```python
from build123d import *

# Parameters (mm, degrees)
F1_DEPTH     = 50
F3_DEPTH     = 45
F4_W         = 15
F4_H         = 40
F5_DEPTH     = 20
F6_T1_DEPTH  = 133.8850999909
F6_T3_DEPTH  = 133.8850999909
F6_T5_DEPTH  = 133.8850999909
F6_T10_DEPTH = 133.8850999909
F6_T15_DEPTH = 133.8850999909
F6_T20_DEPTH = 133.8850999909
F6_T25_DEPTH = 133.8850999909
F6_T30_DEPTH = 133.8850999909


# Not quite as in the source:
# - a fillet or chamfer that OpenCascade refuses, or shapes differently, is made with other operations: its cross-section is extruded or revolved along the edge and cut away or added


with BuildPart() as f1:
    # F0 (on Top) → F1 (new body)
    with BuildSketch(Plane.XY):
        Polygon((29.9990277389, 0.2415258118), (14.7903463808, 26.1006830166), (-15.2086813581, 25.8591572049), (-29.9990277389, -0.2415258118), (-14.7903463808, -26.1006830166), (15.2086813581, -25.8591572049), align=None)
    extrude(amount=F1_DEPTH)

    # F2 (on face) → F3 (cut)
    with BuildSketch(Plane.XY.offset(50)):
        Polygon((24.9981357174, 0.3053041981), (12.2346666673, 21.8016726776), (-12.7634690502, 21.4963684795), (-24.9981357174, -0.3053041981), (-12.2346666673, -21.8016726776), (12.7634690502, -21.4963684795), align=None)
    extrude(amount=-F3_DEPTH, mode=Mode.SUBTRACT)

    # F4 (on face) → F5 (join)
    with BuildSketch(Plane(origin=(0.2091674886, -25.9799201108, 0), x_dir=(0.9999675913, 0.0080508604, 0), z_dir=(0.0080508604, -0.9999675913, 0))):
        with Locations((0, 25)):
            Rectangle(F4_W, F4_H)
    extrude(amount=F5_DEPTH)

    # F6: chamfer of 20 x 5 on 6 edges, made by hand

    # F6_s2 → F6_t1 (cut)
    with BuildSketch(Plane(origin=(33.0034500683, 58.2415425919, 0), x_dir=(0, 0, 1), z_dir=(-0.493011546, -0.8700227672, 0))):
        Polygon((50, 20.9807621135), (30, 25.9807621135), (50, 25.9807621135), align=None)
    extrude(amount=F6_T1_DEPTH, mode=Mode.SUBTRACT)

    # F6_s4 → F6_t3 (cut)
    with BuildSketch(Plane(origin=(66.9403804743, 0.5389451243, 0), x_dir=(0, 0, 1), z_dir=(-0.9999675913, -0.0080508604, 0))):
        Polygon((50, 20.9807621135), (30, 25.9807621135), (50, 25.9807621135), align=None)
    extrude(amount=F6_T3_DEPTH, mode=Mode.SUBTRACT)

    # F6_s6 → F6_t5 (cut)
    with BuildSketch(Plane(origin=(33.936930406, -57.7025974676, 0), x_dir=(0, 0, 1), z_dir=(-0.5069560453, 0.8619719068, 0))):
        Polygon((30, 25.9807621135), (50, 20.9807621135), (50, 25.9807621135), align=None)
    extrude(amount=F6_T5_DEPTH, mode=Mode.SUBTRACT)


with BuildPart() as f6_tool8:
    # F6_s9 → F6_t10 (new body)
    with BuildSketch(Plane(origin=(-33.0034500683, -58.2415425919, 0), x_dir=(0, 0, 1), z_dir=(0.493011546, 0.8700227672, 0))):
        Polygon((30, 25.9807621135), (50, 20.9807621135), (50, 25.9807621135), align=None)
    extrude(amount=F6_T10_DEPTH)

    split(bisect_by=Plane(origin=(7.4997569347, 0.0603814529, 0), x_dir=(0, 0, 1), z_dir=(0.9999675913, 0.0080508604, 0)), keep=Keep.TOP)


with BuildPart() as f1_1:
    add(f1.part)

    # F6_t7: cut F6_tool8
    add(f6_tool8.part, mode=Mode.SUBTRACT)


with BuildPart() as f6_tool13:
    # F6_s14 → F6_t15 (new body)
    with BuildSketch(Plane(origin=(-66.9403804743, -0.5389451243, 0), x_dir=(0, 0, 1), z_dir=(0.9999675913, 0.0080508604, 0))):
        Polygon((30, 25.9807621135), (50, 20.9807621135), (50, 25.9807621135), align=None)
    extrude(amount=F6_T15_DEPTH)

    split(bisect_by=Plane(origin=(-7.4997569347, -0.0603814529, 0), x_dir=(0, 0, 1), z_dir=(-0.9999675913, -0.0080508604, 0)), keep=Keep.TOP)


with BuildPart() as f1_2:
    add(f1_1.part)

    # F6_t12: cut F6_tool13
    add(f6_tool13.part, mode=Mode.SUBTRACT)


with BuildPart() as f6_tool18:
    # F6_s19 → F6_t20 (new body)
    with BuildSketch(Plane(origin=(-66.9403804743, -0.5389451243, 0), x_dir=(0, 0, 1), z_dir=(0.9999675913, 0.0080508604, 0))):
        Polygon((30, 25.9807621135), (50, 20.9807621135), (50, 25.9807621135), align=None)
    extrude(amount=F6_T20_DEPTH)

    split(bisect_by=Plane.XY.offset(45), keep=Keep.TOP)


with BuildPart() as f1_3:
    add(f1_2.part)

    # F6_t17: cut F6_tool18
    add(f6_tool18.part, mode=Mode.SUBTRACT)


with BuildPart() as f6_tool23:
    # F6_s24 → F6_t25 (new body)
    with BuildSketch(Plane(origin=(-66.9403804743, -0.5389451243, 0), x_dir=(0, 0, 1), z_dir=(0.9999675913, 0.0080508604, 0))):
        Polygon((30, 25.9807621135), (50, 20.9807621135), (50, 25.9807621135), align=None)
    extrude(amount=F6_T25_DEPTH)

    split(bisect_by=Plane(origin=(7.4997569347, 0.0603814529, 0), x_dir=(0, 0, 1), z_dir=(0.9999675913, 0.0080508604, 0)), keep=Keep.TOP)


with BuildPart() as f1_4:
    add(f1_3.part)

    # F6_t22: cut F6_tool23
    add(f6_tool23.part, mode=Mode.SUBTRACT)


with BuildPart() as f6_tool28:
    # F6_s29 → F6_t30 (new body)
    with BuildSketch(Plane(origin=(-33.936930406, 57.7025974676, 0), x_dir=(0, 0, 1), z_dir=(0.5069560453, -0.8619719068, 0))):
        Polygon((50, 20.9807621135), (30, 25.9807621135), (50, 25.9807621135), align=None)
    extrude(amount=F6_T30_DEPTH)

    split(bisect_by=Plane(origin=(-7.4997569347, -0.0603814529, 0), x_dir=(0, 0, 1), z_dir=(-0.9999675913, -0.0080508604, 0)), keep=Keep.TOP)


with BuildPart() as f1_5:
    add(f1_4.part)

    # F6_t27: cut F6_tool28
    add(f6_tool28.part, mode=Mode.SUBTRACT)


solid = f1_5.part
```
The listing builds one solid part. Answer for the finished solid, in the listing's coordinates (mm). A direction names the side the tool comes from. Give positions to 0.01 mm unless a question says otherwise; leave off trailing zeros. Order: outer loops, then holes, each group sorted by start corner. A loop starts at its lowest first (then second) coordinate and runs counter-clockwise, first axis right, second up. Notation, with made-up numbers: (15, 65.5) - (59, 65.5) arc R10 ccw to (59, 76.5) - close; hole circle Ø8 at (-27.75, 32.5). An arc over 180 degrees is marked (long way). Answer in a Markdown table with one row per item. Add a question column.
Q1. Which of the six approach directions +Z, -Z, +X, -X, +Y, -Y give full straight-line access (tool end or side, diameter ignored) to faces 4 (the flat face through (-20.586, -11.864, 38.886)), 5 (the flat face through (18.795, -10.748, 26.561))?
Q2. The part is cut by section D-D (z = 8). Determine the outline of the cut face in (x, y), then the cut area to 3 significant figures.
Q3. The part is cut by section C-C (x = -9.5). Determine the outline of the cut face in (y, z) (3 decimals).
Q4. The part is cut by section A-A (z = 44). Determine the outline of the cut face in (x, y).
Q5. Given P1, Ø1, axis at y = -6, z = 39, coming from the +X side; P2, Ø6, axis at y = -16, z = 42, coming from the -X side; P3, Ø10, axis at x = 4.5, y = -11, coming from the +Z side, each flat-ended and moving along its own axis, determine where each tip first touches the part or whether it passes through.
Q6. The part is cut by section B-B (y = 3). Determine the outline of the cut face in (x, z), then the cut area to 3 significant figures.
Q7. Find the intervals of material crossed by line 1 along Z through (x, y) = (-4.5, -38); line 2 along Z through (x, y) = (-13.5, 2.5); line 3 along X through (y, z) = (19.5, 22), in increasing order. Write a range as [from, to].
Q8. For a pull along X with two mould halves and no side action, classify faces 1 (the flat face through (0, -36, 5)), 2 (the flat face through (-18.795, 10.748, 26.561)), 3 (the flat face through (20.62, -11.93, 38.64)) as released by +X, released by -X, zero draft, split by the parting line, or undercut.
Determined:
| question | item | result |
|---|---|---|
| 1 | face 4 | +Z, -X, -Y |
| 1 | face 5 | +Z |
| 2 | outline | (-30, -0.24) - (-14.79, -26.1) - (-7.29, -26.04) - (-7.13, -46.04) - (7.87, -45.92) - (7.71, -25.92) - (15.21, -25.86) - (30, 0.24) - (14.79, 26.1) - (-15.21, 25.86) - close; hole (-25, -0.31) - (-12.23, -21.8) - (12.76, -21.5) - (25, 0.31) - (12.23, 21.8) - (-12.76, 21.5) - close |
| 2 | area | 1,010 mm² |
| 3 | outline | (-26.058, 0) - (25.905, 0) - (25.905, 30) - (21.536, 47.475) - (21.536, 5) - (-21.768, 5) - (-21.768, 47.159) - (-26.058, 30) - close |
| 4 | outline | (-25.96, -0.21) - (-12.8, -22.58) - (-7.32, -22.54) - (-7.13, -46.04) - (7.87, -45.92) - (7.68, -22.42) - (13.16, -22.38) - (25.96, 0.21) - (12.8, 22.58) - (-13.16, 22.38) - close; hole (-25, -0.31) - (-12.23, -21.8) - (12.76, -21.5) - (25, 0.31) - (12.23, 21.8) - (-12.76, 21.5) - close |
| 5 | P1 | stops at x = 24.19 |
| 5 | P2 | stops at x = -19.22 |
| 5 | P3 | stops at z = 5 |
| 6 | outline | (-28.16, 0) - (28.38, 0) - (28.38, 30) - (23.4, 47.17) - (23.4, 5) - (-23.14, 5) - (-23.14, 47.47) - (-28.16, 30) - close |
| 6 | area | 619 mm² |
| 7 | line 1 | z = [5, 45] |
| 7 | line 2 | z = [0, 5] |
| 7 | line 3 | x = [-18.81, -13.88], [13.6, 18.67] |
| 8 | face 1 | zero draft |
| 8 | face 2 | undercut |
| 8 | face 3 | released by +X |
